```python
from build123d import *

# Parameters (mm, degrees)
ESTRUSIONE_ESTRUSIONE1_DEPTH = 5
FORO_PER_VITE_M3_1_D         = 3.4
RIPETIZIONECIRCOLARE1_COUNT  = 4
SCHIZZO4_W                   = 45
SCHIZZO4_H                   = 45
ESTRUSIONE_ESTRUSIONE2_DEPTH = 103.8
SCHIZZO5_W                   = 41
SCHIZZO5_H                   = 41
TAGLIO_ESTRUSIONE1_DEPTH     = 117.779450247
TAGLIO_ESTRUSIONE2_REACH     = 126.474
SCHIZZO6_W                   = 30
SCHIZZO6_H                   = 93.8
SCHIZZO7_W                   = 45
SCHIZZO7_H                   = 45
ESTRUSIONE_ESTRUSIONE3_DEPTH = 10
JOINT_MOTOR_HOUSING_D        = 3.4
RIPETIZIONECIRCOLARE2_COUNT  = 4
JOINT_MOTOR_ARM_D            = 5.5


with BuildPart() as part:
    # Schizzo1 → Estrusione-Estrusione1 (new body)
    with BuildSketch(Plane(origin=(0, 0, 0), x_dir=(0, 1, 0), z_dir=(0, 0, 1))):
        Polygon((-22.5, 22.5), (-30, 0), (-22.5, -22.5), (0, -30), (22.5, -22.5), (30, 0), (22.5, 22.5), (0, 30), align=None)
    extrude(amount=-ESTRUSIONE_ESTRUSIONE1_DEPTH)

    # Foro per Vite M3-1 (through all)
    with Locations(Plane.XY):
        with Locations((-25, 0)):
            foro_per_vite_m3_1 = Hole(FORO_PER_VITE_M3_1_D / 2)

    # RipetizioneCircolare1: Foro per Vite M3-1 ×4 about axis
    ripetizionecircolare1_axis = Axis((0.084350334, 0, 0), (0, 0, 1))
    for i in range(1, RIPETIZIONECIRCOLARE1_COUNT):
        add(foro_per_vite_m3_1.rotate(ripetizionecircolare1_axis, i * 360 / RIPETIZIONECIRCOLARE1_COUNT), mode=Mode.SUBTRACT)

    # Schizzo4 → Estrusione-Estrusione2 (add)
    with BuildSketch(Plane(origin=(0, 0, -5), x_dir=(1, 0, 0), z_dir=(0, 0, -1))):
        Rectangle(SCHIZZO4_W, SCHIZZO4_H)
    extrude(amount=ESTRUSIONE_ESTRUSIONE2_DEPTH)

    # Schizzo5 → Taglio-Estrusione1 (cut, through all)
    with BuildSketch(Plane(origin=(0, 0, -108.8), x_dir=(1, 0, 0), z_dir=(0, 0, -1))):
        Rectangle(SCHIZZO5_W, SCHIZZO5_H)
    extrude(amount=-TAGLIO_ESTRUSIONE1_DEPTH, mode=Mode.SUBTRACT)

    # Schizzo6 → Taglio-Estrusione2 (cut, up to next)
    with BuildSketch(Plane.YZ.offset(22.5), mode=Mode.PRIVATE) as taglio_estrusione2_sk1:
        with Locations((0, -61.9)):
            Rectangle(SCHIZZO6_W, SCHIZZO6_H)
    taglio_estrusione2_tool1 = extrude(taglio_estrusione2_sk1.sketch, amount=-TAGLIO_ESTRUSIONE2_REACH, mode=Mode.PRIVATE) & part.part
    add(taglio_estrusione2_tool1.solids().sort_by_distance((22.5, 0, -61.9))[0], mode=Mode.SUBTRACT)

    # Schizzo7 → Estrusione-Estrusione3 (add)
    with BuildSketch(Plane(origin=(0, 0, -108.8), x_dir=(1, 0, 0), z_dir=(0, 0, -1))):
        Rectangle(SCHIZZO7_W, SCHIZZO7_H)
    extrude(amount=ESTRUSIONE_ESTRUSIONE3_DEPTH)

    # Joint-motor-housing (through all)
    with Locations(Plane(origin=(0, 0, -118.8), x_dir=(-1, 0, 0), z_dir=(0, 0, -1))):
        with Locations((15.52, 15.52)):
            joint_motor_housing = Hole(JOINT_MOTOR_HOUSING_D / 2)

    # RipetizioneCircolare2: Joint-motor-housing ×4 about axis
    ripetizionecircolare2_axis = Axis((0.069898196, -0.069898196, 0), (0, 0, 1))
    for i in range(1, RIPETIZIONECIRCOLARE2_COUNT):
        add(joint_motor_housing.rotate(ripetizionecircolare2_axis, i * 360 / RIPETIZIONECIRCOLARE2_COUNT), mode=Mode.SUBTRACT)

    # Joint-motor-arm (through all)
    with Locations(Plane(origin=(0, 0, -118.8), x_dir=(-1, 0, 0), z_dir=(0, 0, -1))):
        with Locations((0, 0)):
            Hole(JOINT_MOTOR_ARM_D / 2)


solid = part.part
```
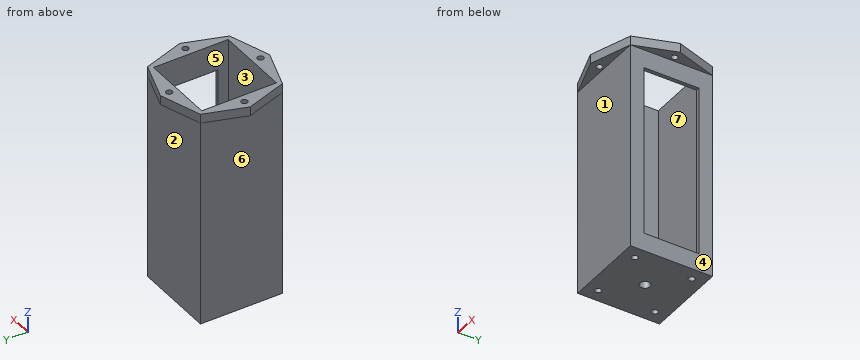
Geometry: final body of the model. Coordinates: model frame, mm. Face numbers are marked on the shaded views. A direction names the side the tool comes from. Coordinates: 2 decimals unless noted, no trailing zeros. Order: outer loops, then holes, each group sorted by start corner. A loop starts at its lowest first (then second) coordinate and runs counter-clockwise, first axis right, second up. Notation, with made-up numbers: (-1.75, -12) -> (49.25, -12) arc R36 cw to (49.25, 26) -> close; hole circle Ø6 at (5.25, 16.25). An arc over 180 degrees is marked (long way). Answer in a Markdown table with one row per item.
Item 1: Ray query, L1, parallel to Y at x = -4, z = -59; L2, parallel to Y at x = 0, z = -115.75. Return the intervals inside material, ascending.
Return value:
| item | result |
|---|---|
| L1 | y = -22.5 to -20.5, 20.5 to 22.5 |
| L2 | y = -22.5 to -2.75, 2.75 to 22.5 |
Item 2: Section A-A on x = -25. Output: boundary loops of the cut face in (y, z).
Return value:
| item | result |
|---|---|
| outline | (-15, -5) -> (-1.7, -5) -> (-1.7, 0) -> (-15, 0) -> close; (1.7, -5) -> (15, -5) -> (15, 0) -> (1.7, 0) -> close |
Item 3: Section B-B on y = 9. Output: boundary loops of the cut face in (x, z), plus the area to 3 significant figures.
Return value:
| item | result |
|---|---|
| outline | (-27, -5) -> (-22.5, -5) -> (-22.5, -118.8) -> (22.5, -118.8) -> (22.5, -108.8) -> (-20.5, -108.8) -> (-20.5, 0) -> (-27, 0) -> close; (20.5, -15) -> (22.5, -15) -> (22.5, -5) -> (27, -5) -> (27, 0) -> (20.5, 0) -> close |
| area | 743 mm² |
Item 4: Section C-C on z = -58. Output: boundary loops of the cut face in (x, y), plus the area to 3 significant figures.
Return value:
| item | result |
|---|---|
| outline | (-22.5, -22.5) -> (22.5, -22.5) -> (22.5, -15) -> (20.5, -15) -> (20.5, -20.5) -> (-20.5, -20.5) -> (-20.5, 20.5) -> (20.5, 20.5) -> (20.5, 15) -> (22.5, 15) -> (22.5, 22.5) -> (-22.5, 22.5) -> close |
| area | 284 mm² |
Item 5: Draft query along X for the marked faces 4, 5, 6 and 7. Return one class per face: released by +X, released by -X, zero draft, split by the parting line, or undercut.
Return value:
| item | result |
|---|---|
| face 4 | released by +X |
| face 5 | undercut |
| face 6 | released by -X |
| face 7 | undercut |
Item 6: Contact query for flat-ended pins moving along their axis: P1, Ø13.5, axis at x = -3.5, z = -69, coming from the +Y side; P2, Ø2, axis at x = 27.5, y = -5, coming from the -Z side; P3, Ø2.5, axis at x = 15.66, y = 15.52, coming from the -Z side; P4, Ø2, axis at x = 15, y = -5, coming from the +Z side. Output: stop coordinate, or through.
Return value:
| item | result |
|---|---|
| P1 | stops at y = 22.5 |
| P2 | stops at z = -5 |
| P3 | passes through |
| P4 | stops at z = -108.8 |
Item 7: Section D-D on x = -15.52. Output: boundary loops of the cut face in (y, z), plus the area to 3 significant figures.
Return value:
| item | result |
|---|---|
| outline | (-24.83, -5) -> (-22.5, -5) -> (-22.5, -118.8) -> (-17.36, -118.8) -> (-17.36, -108.8) -> (-20.5, -108.8) -> (-20.5, 0) -> (-24.83, 0) -> close; (-13.96, -118.8) -> (13.82, -118.8) -> (13.82, -108.8) -> (-13.96, -108.8) -> close; (17.22, -118.8) -> (22.5, -118.8) -> (22.5, -5) -> (24.83, -5) -> (24.83, 0) -> (20.5, 0) -> (20.5, -108.8) -> (17.22, -108.8) -> close |
| area | 840 mm² |
Item 8: Access query for the marked faces 1, 2 and 3. Directions: +Z, -Z, +X, -X, +Y, -Y. A direction counts if a zero-diameter tool reaches every point of the face in a straight line with its end or side. Return the directions, or none.
Return value:
| item | result |
|---|---|
| face 1 | -Z, +X, -X, -Y |
| face 2 | -Z, +X, -X, +Y |
| face 3 | +Z |
